Verification items for the finished model (mm, model axes). A direction names the side the tool comes from. Give positions to 0.01 mm unless a question says otherwise; leave off trailing zeros. Write each loop counter-clockwise with the first axis right and the second up, starting at its lowest first coordinate (ties: lowest second). Pieces come first, ordered by that corner, then holes. Notation, with made-up numbers: (8.5, 14) -> (42.5, 14) arc R18 ccw to (42.5, 27) -> close; hole circle Ø5 at (77.5, -30.75). An arc over 180 degrees is marked (long way). Answer as CSV lines item,"result". Start each with the question number.
1) Sectioned sample at D-D on z = 0.65. Give the number of separate pieces and of enclosed holes in the cut face, and give its area (3 significant figures).
2) Gauge pin test, flat end, axial feed: pin 1 Ø1.6 at (x, z) = (-14, 1.5) entering from +Y. Record the tip position at first contact, or that the pin passes through.
3) Mould release check, pull along X, two halves, no side actions. Record for faces 4 (the flat face through (14, 3.248, 2)), 5 (the flat face through (0, 9, 3.18)), 6 (the flat face through (-17.5, 0, 2)): released by +X, released by -X, zero draft, split by the parting line, or undercut.
4) Sectioned sample at A-A on x = -6. Record the cut outline in (y, z), and give its area (3 significant figures).
5) Material ranges on L1, parallel to Y at x = 13.63, z = 1.4; L2, parallel to Y at x = 0.5, z = 0.1; L3, parallel to X at y = 11, z = 1.1, recorded low to high.
6) Sectioned sample at B-B on y = 4.5. Record the cut outline in (x, z).
7) Tool access check on faces 1 (the flat face through (-15.5, 10.368, 1.6)), 2 (the flat face through (13, 11, 2)), 3 (the flat face through (0, 9, 0)). Record the directions out of +Z, -Z, +X, -X, +Y, -Y that give a thin tool (end or side, any length) a straight path to the whole face; none if there is none.
8) Sectioned sample at C-C on y = 1.75. Record the cut outline in (x, z), and give its area (4 significant figures).
```python
from build123d import *

# Parameters (mm, degrees)
SKETCH1_W           = 35
SKETCH1_H           = 25
BOSS_EXTRUDE1_DEPTH = 3.18
SKETCH2_W           = 22.5
SKETCH2_H           = 12
CUT_EXTRUDE1_DEPTH  = 3.18
SKETCH3_R           = 1
CUT_EXTRUDE2_DEPTH  = 3.18
CUT_EXTRUDE4_DEPTH  = 3.18


with BuildPart() as part:
    # Sketch1 → Boss-Extrude1 (new body)
    with BuildSketch(Plane.XY):
        Rectangle(SKETCH1_W, SKETCH1_H)
    extrude(amount=BOSS_EXTRUDE1_DEPTH)

    # Sketch2 → Cut-Extrude1 (cut)
    with BuildSketch(Plane.XY.offset(3.18)):
        Rectangle(SKETCH2_W, SKETCH2_H)
    extrude(amount=-CUT_EXTRUDE1_DEPTH, mode=Mode.SUBTRACT)

    # Sketch3 → Cut-Extrude2 (cut)
    with BuildSketch(Plane.XY.offset(3.18)):
        with Locations((-13.63, 0)):
            Circle(SKETCH3_R)
    cut_extrude2 = extrude(amount=-CUT_EXTRUDE2_DEPTH, mode=Mode.SUBTRACT)

    # Mirror1: Cut-Extrude2 across plane
    add(cut_extrude2.mirror(Plane(origin=(0, 0, 0), x_dir=(0, 0, 1), z_dir=(1, 0, 0))), mode=Mode.SUBTRACT)

    # Sketch5 → Cut-Extrude4 (cut)
    with BuildSketch(Plane.XY.offset(3.18)):
        Polygon((-13, 12.5), (-15, 12.5), (-15, 10.368), (-16, 10.368), (-16, 9.248), (-15, 9.248), (-15, 3.248), (-13, 3.248), (-13, 9.248), (-12, 9.248), (-12, 10.368), (-13, 10.368), align=None)
    cut_extrude4 = extrude(amount=-CUT_EXTRUDE4_DEPTH, mode=Mode.SUBTRACT)

    # Mirror2: Cut-Extrude4 across plane
    add(cut_extrude4.mirror(Plane(origin=(0, 0, 0), x_dir=(0, 0, 1), z_dir=(1, 0, 0))), mode=Mode.SUBTRACT)


solid = part.part
```
Ans:
1,separate pieces,"1"
1,enclosed holes,"3"
1,area,"557 mm²"
2,pin 1,"stops at y = 3.25"
3,face 4,"undercut"
3,face 5,"zero draft"
3,face 6,"released by -X"
4,outline,"(-12.5, 0) -> (-6, 0) -> (-6, 3.18) -> (-12.5, 3.18) -> close; (6, 0) -> (12.5, 0) -> (12.5, 3.18) -> (6, 3.18) -> close"
4,area,"41.3 mm²"
5,L1,"y = -12.5 to -1, 1 to 3.25"
5,L2,"y = -12.5 to -6, 6 to 12.5"
5,L3,"x = -17.5 to -15, -13 to 13, 15 to 17.5"
6,outline,"(-17.5, 0) -> (-15, 0) -> (-15, 3.18) -> (-17.5, 3.18) -> close; (-13, 0) -> (-11.25, 0) -> (-11.25, 3.18) -> (-13, 3.18) -> close; (11.25, 0) -> (13, 0) -> (13, 3.18) -> (11.25, 3.18) -> close; (15, 0) -> (17.5, 0) -> (17.5, 3.18) -> (15, 3.18) -> close"
7,face 1,"+Z, -Z"
7,face 2,"+Z, -Z, +Y"
7,face 3,"-Z, +X, -X, +Y, -Y"
8,outline,"(-17.5, 0) -> (-11.25, 0) -> (-11.25, 3.18) -> (-17.5, 3.18) -> close; (11.25, 0) -> (17.5, 0) -> (17.5, 3.18) -> (11.25, 3.18) -> close"
8,area,"39.75 mm²"
